from build123d import *

# Parameters (mm, degrees)
F0_R     = 60
F0_R_2   = 58.5
F1_DEPTH = 70
F2_R     = 60
F3_DEPTH = 25
F4_R     = 35.1
F5_R     = 60
F6_DEPTH = 117.5
F7_R     = 60
F8_W     = 33.7252318859
F8_H     = 51.0791689157
F9_DEPTH = 133


with BuildPart() as f1:
    # F0 (on Top) → F1 (new body)
    with BuildSketch(Plane.XY):
        Circle(F0_R)
        Circle(F0_R_2, mode=Mode.SUBTRACT)
    extrude(amount=-F1_DEPTH)

    # F2 (on Top) → F3 (join)
    with BuildSketch(Plane.XY):
        Circle(F2_R)
    extrude(amount=F3_DEPTH)

    # F4
    f4_edges = [f1.edges().sort_by_distance(p)[0] for p in [
        (-60, 0, 25),
    ]]
    fillet(f4_edges, radius=F4_R)

    # F5 (on Top) → F6 (join)
    with BuildSketch(Plane.XY):
        Circle(F5_R)
    extrude(amount=-F6_DEPTH)

    # F7
    f7_edges = [f1.edges().sort_by_distance(p)[0] for p in [
        (-60, 0, -117.5),
        (-24.9, 0, 25),
    ]]
    fillet(f7_edges, radius=F7_R)

    # F8 (on Top) → F9 (cut)
    with BuildSketch(Plane.XY):
        with Locations((47.9409359396, 0.4799189046)):
            Rectangle(F8_W, F8_H)
    extrude(amount=-F9_DEPTH, mode=Mode.SUBTRACT)


solid = f1.part
The listing builds one solid part. Answer for the finished solid, in the listing's coordinates (mm). A direction names the side the tool comes from. Round coordinates to 2 decimals unless told otherwise and drop trailing zeros. Loops run counter-clockwise (first coordinate to the right, second up) from the corner with the lowest first, then second, coordinate; pieces in that order, holes last. Notation, with made-up numbers: M 29.25,76 L 64.25,76 A15 ccw 64.25,93 Z; hole C 27,82 d7. An arc over 180 degrees is marked long. Return JSON: item names as keys, results as strings.
Q1. Each of these flat-tipped pins is pushed along its axis until it touches: pin 1 Ø5 at (x, z) = (42, -41.5) entering from +Y; pin 2 Ø12 at (y, z) = (28, -51.5) entering from -X; pin 3 Ø10 at (y, z) = (-23.5, -87) entering from -X. Where does it stop, or does it pass through?
Results list:
{"pin 1": "stops at y = 45.16", "pin 2": "stops at x = -55.82", "pin 3": "stops at x = -50.3"}
Q2. Find section A-A, the plane z = -28. Determine the outline of the cut face in (x, y).
Results list:
{"outline": "M 31.08,-25.06 L 31.08,26.02 L 54.06,26.02 A60 ccw long 54.52,-25.06 Z"}
Q3. Find the intervals of material crossed by line 1 along X through (y, z) = (1.5, -26.5); line 2 along Y through (x, z) = (45, -37); line 3 along X through (y, z) = (-17.5, -8), in increasing order. Write a range as from..to.
Results list:
{"line 1": "x = -59.98..31.08", "line 2": "y = -39.69..-25.06, 26.02..39.69", "line 3": "x = -57.39..31.08"}
Q4. Which of the six approach directions +Z, -Z, +X, -X, +Y, -Y give full straight-line access (tool end or side, diameter ignored) to faces 1 (the face through (10, 58, 0)), 2 (the face through (45, 1, 0))?
Results list:
{"face 1": "+Z", "face 2": "-Z, +X"}
Q5. The mould has two halves that part along Y. Classify faces 3 (the face through (42, 26.02, -50)), 4 (the face through (-59.975, 1.739, -28.348)), 5 (the face through (0, 0, 25)): released by +Y, released by -Y, zero draft, split by the parting line, or undercut.
Results list:
{"face 3": "undercut", "face 4": "split by the parting line", "face 5": "zero draft"}
